The listing builds one solid part. Answer for the finished solid, in the listing's coordinates (mm). Face numbers are marked on the shaded views. Coordinates: 2 decimals unless noted, no trailing zeros. Loops run counter-clockwise (first coordinate to the right, second up) from the corner with the lowest first, then second, coordinate; pieces in that order, holes last. Notation, with made-up numbers: (51.5, 61.5) - (96.5, 61.5) arc R29 ccw to (96.5, 92.5) - close; hole circle Ø6 at (48.5, -6). An arc over 180 degrees is marked (long way). Return JSON: item names as keys, results as strings. Group by question number.
1. The mould has two halves that part along Y. Classify the marked faces 1, 2, 3 and 4: pulls with the +Y half, pulls with the -Y half, needs draft (parallel to the pull), parting line crosses it, or undercut.
2. Section D-D (x = 7.5) is taken. Write down the section's boundary in (y, z).
3. Each of these flat-tipped pins is pushed along its axis until it touches: P1, Ø7.5, axis at x = 59.5, y = 9, coming from the -Z side; P2, Ø7.5, axis at x = 27.5, y = 8, coming from the +Z side; P3, Ø24, axis at x = 109, z = 5, coming from the -Y side; P4, Ø1, axis at x = 41.5, y = -24, coming from the +Z side. Where does it stop, or does it pass through?
4. Section C-C (z = -3) is taken. Write down the section's boundary in (x, y), and give its area (3 significant figures).
5. Find the intervals of material crossed by line 1 along X through (y, z) = (7.5, 4.1); line 2 along X through (y, z) = (-23, 22); line 3 along Y through (x, z) = (97.5, 3.8), in increasing order.
6. Section A-A (y = 7.5) is taken. Write down the section's boundary in (x, z).
7. Section B-B (x = 53) is taken. Write down the section's boundary in (y, z).
```python
from build123d import *

# Parameters (mm, degrees)
F1_DEPTH       = 105
F3_R           = 2
F4_D           = 3.3
F4_DEPTH       = 15
F4_CSINK_D     = 6.72
F4_CSINK_ANGLE = 90
F4_TIP         = 0.9914200214
F6_D           = 3.3
F6_DEPTH       = 15
F6_TIP         = 0.9914200214
F7_W           = 20
F7_H           = 3.8302222156
F8_DEPTH       = 25
F9_R           = 5
F11_DEPTH      = 0.22


with BuildPart() as f1:
    # F0 (on Right) → F1 (new body)
    with BuildSketch(Plane.YZ):
        Polygon((-11.4906666468, 9.6418141453), (0, 0), (15, 0), (15, 5), (0, 5), (-9.0286472643, 12.5759345895), align=None)
    extrude(amount=F1_DEPTH)

    # F3
    f3_edges = [f1.edges().sort_by_distance(p)[0] for p in [
        (0, 15, 2.5),
        (105, 15, 2.5),
        (105, -10.259657, 11.108874),
        (0, -10.259657, 11.108874),
    ]]
    fillet(f3_edges, radius=F3_R)

    # F4
    with Locations(Plane(origin=(0, 0, 0), x_dir=(1, 0, 0), z_dir=(0, 0, -1))):
        with Locations((7.5, -7.5), (97.5, -7.5)):
            CounterSinkHole(F4_D / 2, F4_CSINK_D / 2, depth=F4_DEPTH, counter_sink_angle=F4_CSINK_ANGLE)
            with Locations((0, 0, -(F4_DEPTH + F4_TIP / 2))):  # 118° drill point
                Cone(0, F4_D / 2, F4_TIP, mode=Mode.SUBTRACT)

    # F6
    with Locations(Plane(origin=(0, 0, 0), x_dir=(1, 0, 0), z_dir=(0, -0.6427876097, -0.7660444431))):
        with Locations((17.5, 7.5), (87.5, 7.5)):
            Hole(F6_D / 2, depth=F6_DEPTH)
            with Locations((0, 0, -(F6_DEPTH + F6_TIP / 2))):  # 118° drill point
                Cone(0, F6_D / 2, F6_TIP, mode=Mode.SUBTRACT)

    # F7 (on face) → F8 (join)
    with BuildSketch(Plane(origin=(0, -11.4906666468, 9.6418141453), x_dir=(1, 0, 0), z_dir=(0, -0.7660444431, 0.6427876097))):
        with Locations((52.5, 1.9151111078)):
            Rectangle(F7_W, F7_H)
    extrude(amount=F8_DEPTH)

    # F9
    f9_edges = [f1.edges().sort_by_distance(p)[0] for p in [
        (42.5, -10.259657, 11.108874),
        (62.5, -10.259657, 11.108874),
        (62.5, -29.410768, 27.178565),
        (42.5, -29.410768, 27.178565),
    ]]
    fillet(f9_edges, radius=F9_R)

    # F10 (on face) → F11 (join)
    with BuildSketch(Plane(origin=(0, 15, 0), x_dir=(-1, 0, 0), z_dir=(0, 1, 0))):
        with BuildLine():
            ThreePointArc((13, 2.5), (-0.7456060958, 17.4474578418), (-16.7901994577, 5))
            Line((-16.7901994577, 5), (-2, 5))
            Line((-2, 5), (-2, 0))
            Line((-2, 0), (-16.7901994577, 0))
            ThreePointArc((-16.7901994577, 0), (-0.7456060958, -12.4474578418), (13, 2.5))
        make_face()
        with BuildLine():
            Line((-103, 5), (-88.2098005423, 5))
            ThreePointArc((-88.2098005423, 5), (-118, 2.5), (-88.2098005423, 0))
            Line((-88.2098005423, 0), (-103, 0))
            Line((-103, 0), (-103, 5))
        make_face()
    extrude(amount=-F11_DEPTH)


solid = f1.part
```
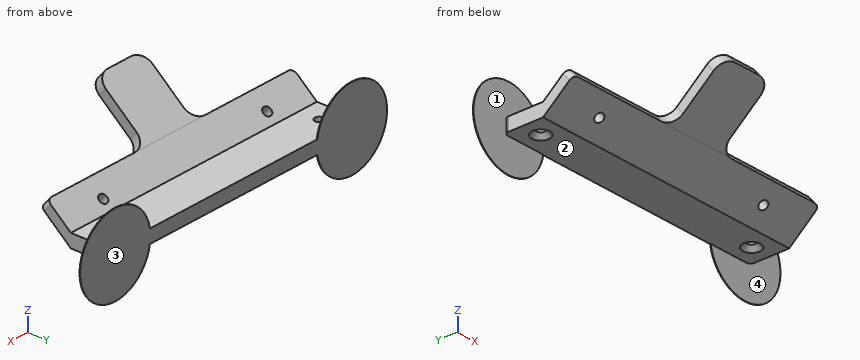
The answers:
{
 "1": {"face 1": "undercut", "face 2": "needs draft", "face 3": "pulls with the +Y half", "face 4": "undercut"},
 "2": {"outline": "(-11.49, 9.64) - (0, 0) - (4.14, 0) - (5.85, 1.71) - (5.85, 5) - (0, 5) - (-9.03, 12.58) - close; (9.15, 1.71) - (10.86, 0) - (14.78, 0) - (14.78, -11.46) - (15, -11.46) - (15, 16.46) - (14.78, 16.46) - (14.78, 5) - (9.15, 5) - close"},
 "3": {"P1": "stops at z = 0", "P2": "stops at z = 5", "P3": "stops at y = -11.49", "P4": "passes through"},
 "4": {"outline": "(-11.96, 14.78) - (15.96, 14.78) - (15.96, 15) - (-11.96, 15) - close; (89.04, 14.78) - (116.96, 14.78) - (116.96, 15) - (89.04, 15) - close", "area": "12.3 mm2"},
 "5": {"line 1": "x = 0 to 5.85, 9.15 to 95.85, 99.15 to 105", "line 2": "x = 42.5 to 62.5", "line 3": "y = -4.53 to 5.85, 9.15 to 15"},
 "6": {"outline": "(0, 0) - (4.14, 0) - (5.85, 1.71) - (5.85, 5) - (0, 5) - close; (9.15, 1.71) - (10.86, 0) - (94.14, 0) - (95.85, 1.71) - (95.85, 5) - (9.15, 5) - close; (99.15, 1.71) - (100.86, 0) - (105, 0) - (105, 5) - (99.15, 5) - close"},
 "7": {"outline": "(-30.64, 25.71) - (0, 0) - (15, 0) - (15, 5) - (0, 5) - (-28.18, 28.65) - close"}
}
